Can you work these out from the model? Positions are in its coordinate system, mm. A direction names the side the tool comes from. Coordinates: 2 decimals unless noted, no trailing zeros. Order: outer loops, then holes, each group sorted by start corner. A loop starts at its lowest first (then second) coordinate and runs counter-clockwise, first axis right, second up. Notation, with made-up numbers: (4.5, -35) -> (36.5, -35) arc R17 ccw to (36.5, -27) -> close; hole circle Ø4 at (44.25, 61.5). An arc over 180 degrees is marked (long way). Use a Markdown table: item, result. Add a question column.
1. We'd pull the mould along Z, two halves only. Please class faces 1 (the flat face through (10, 0, 0)), 2 (the flat face through (7.535, 14.93, 1.479)), 3 (the flat face through (5, 0, 3)): pulls with the +Z half, pulls with the -Z half, needs draft (parallel to the pull), parting line crosses it, or undercut.
2. For pin 1 Ø2.5 at (x, z) = (-12.5, 15) entering from -Y, with a flat end and sliding along its axis, tell me the tip position at first contact or that it passes through.
3. Suppose I cut it at B-B, the plane z = 17. List the corners of the cut face in (x, y) for me.
4. If I drill on line 1 along Z through (x, y) = (24.5, -9.5); line 2 along X through (y, z) = (1.5, 5.75); line 3 along Y through (x, z) = (16, 25.25), over which ranges is the centre line in solid material (lowest first)? Write a range as from..to.
5. Suppose I cut it at A-A, the plane y = 0. List the corners of the cut face in (x, z) for me, then the cut area to 3 significant figures.
6. Suppose I cut it at D-D, the plane y = -9. List the corners of the cut face in (x, z) for me.
7. Suppose I cut it at C-C, the plane x = 8. List the corners of the cut face in (y, z) for me, then the cut area to 3 significant figures.
8. For faces 4 (the flat face through (-10, 0, 13)), 5 (the flat face through (31, -10, 13)), 6 (the cylindrical face through (-0.54, 10.06, 24.48)), which set-ups out of +Z, -Z, +X, -X, +Y, -Y let a thin tool reach every point of the face, with its end or its side?
```python
from build123d import *

# Parameters (mm, degrees)
F0_R        = 2.75
F0_W        = 20
F0_H        = 20
F1_DEPTH    = 3
F0_W_2      = 5
F2_DEPTH    = 26
F3_START    = 20
F1_FACE_R   = 2.75
F1_FACE_R_2 = 2.5
F3_DEPTH    = 3


with BuildPart() as f1:
    # F0 (on Top) → F1 (new body)
    with BuildSketch(Plane.XY):
        Polygon((0, 10), (-10, 10), (-10, -10), (0, -10), (10, -10), (10, 10), align=None)
        with Locations((-5, 0)):
            Circle(F0_R, mode=Mode.SUBTRACT)
        Polygon((0, -10), (-10, -10), (-5, -20), (5, -20), (10, -10), align=None)
        with BuildLine():
            ThreePointArc((2.5, -12.5), (-1.767766953, -14.267766953), (0, -10))
            ThreePointArc((0, -10), (1.767766953, -10.732233047), (2.5, -12.5))
        make_face(mode=Mode.SUBTRACT)
        Polygon((-5, 20), (-10, 10), (0, 10), (10, 10), (5, 20), align=None)
        with BuildLine():
            ThreePointArc((2.5, 12.5), (1.767766953, 10.732233047), (0, 10))
            ThreePointArc((0, 10), (-1.767766953, 14.267766953), (2.5, 12.5))
        make_face(mode=Mode.SUBTRACT)
        with Locations((20, 0)):
            Rectangle(F0_W, F0_H)
        with Locations((25, 0)):
            Circle(F0_R, mode=Mode.SUBTRACT)
    extrude(amount=F1_DEPTH)

    # F0 (on Top) → F2 (join)
    with BuildSketch(Plane.XY):
        with Locations((-12.5, 0)):
            Rectangle(F0_W_2, F0_H)
        with Locations((32.5, 0)):
            Rectangle(F0_W_2, F0_H)
    extrude(amount=F2_DEPTH)

    # F1_face (on face) → F3 (join)
    with BuildSketch(Plane(origin=(7.4267013707, 0, 3), x_dir=(1, 0, 0), z_dir=(0, 0, 1)).offset(F3_START)):
        Polygon((-17.4267013707, 10), (-17.4267013707, -10), (-12.4267013707, -20), (-2.4267013707, -20), (2.5732986293, -10), (22.5732986293, -10), (22.5732986293, 10), (2.5732986293, 10), (-2.4267013707, 20), (-12.4267013707, 20), align=None)
        with Locations((-12.4267013707, 0)):
            Circle(F1_FACE_R, mode=Mode.SUBTRACT)
        with Locations((-7.4267013707, -12.5)):
            Circle(F1_FACE_R_2, mode=Mode.SUBTRACT)
        with Locations((-7.4267013707, 12.5)):
            Circle(F1_FACE_R_2, mode=Mode.SUBTRACT)
        with Locations((17.5732986293, 0)):
            Circle(F1_FACE_R, mode=Mode.SUBTRACT)
    extrude(amount=F3_DEPTH)


solid = f1.part
```
Worked out:
| question | item | result |
|---|---|---|
| 1 | face 1 | pulls with the -Z half |
| 1 | face 2 | needs draft |
| 1 | face 3 | undercut |
| 2 | pin 1 | stops at y = -10 |
| 3 | outline | (-15, -10) -> (-10, -10) -> (-10, 10) -> (-15, 10) -> close; (30, -10) -> (35, -10) -> (35, 10) -> (30, 10) -> close |
| 4 | line 1 | z = 0..3, 23..26 |
| 4 | line 2 | x = -15..-10, 30..35 |
| 4 | line 3 | y = -10..10 |
| 5 | outline | (-15, 0) -> (-7.75, 0) -> (-7.75, 3) -> (-10, 3) -> (-10, 23) -> (-7.75, 23) -> (-7.75, 26) -> (-15, 26) -> close; (-2.25, 0) -> (22.25, 0) -> (22.25, 3) -> (-2.25, 3) -> close; (-2.25, 23) -> (22.25, 23) -> (22.25, 26) -> (-2.25, 26) -> close; (27.75, 0) -> (35, 0) -> (35, 26) -> (27.75, 26) -> (27.75, 23) -> (30, 23) -> (30, 3) -> (27.75, 3) -> close |
| 5 | area | 434 mm² |
| 6 | outline | (-15, 0) -> (35, 0) -> (35, 26) -> (-15, 26) -> close; hole (-10, 3) -> (30, 3) -> (30, 23) -> (-10, 23) -> close |
| 7 | outline | (-14, 0) -> (14, 0) -> (14, 3) -> (-14, 3) -> close; (-14, 23) -> (14, 23) -> (14, 26) -> (-14, 26) -> close |
| 7 | area | 168 mm² |
| 8 | face 4 | +Y, -Y |
| 8 | face 5 | +Z, -Z, +X, -Y |
| 8 | face 6 | +Z, -Z |
